Can you work these out from the model? Positions are in its coordinate system, mm. Coordinates: 2 decimals unless noted, no trailing zeros. Order: outer loops, then holes, each group sorted by start corner. A loop starts at its lowest first (then second) coordinate and runs counter-clockwise, first axis right, second up. Notation, with made-up numbers: (-11, 41.25) -> (17, 41.25) arc R31 cw to (17, 71.25) -> close; hole circle Ø7 at (50.25, -8). An arc over 180 degrees is marked (long way). Answer in a Markdown table with one row per item. Add a question column.
1. Imagine slicing it at C-C on z = 1.5. State how many separate pieces and enclosed holes the cut face has, plus the area to 3 significant figures.
2. If I drill on line 1 along Y through (x, z) = (-21, 3.5); line 2 along Y through (x, z) = (-10.5, 5); line 3 along Y through (x, z) = (-76.2, 3.75), over which ranges is the centre line in solid material (lowest first)? Write a range as [from, to].
3. We'd pull the mould along X, two halves only. Please class faces 1 (the face through (-62.396, 55.247, 3.131)), 2 (the face through (-77.12, 137.48, 3.13)), 3 (the face through (66, 42, 0)): pulls with the +X half, pulls with the -X half, needs draft (parallel to the pull), parting line crosses it, or undercut.
4. Imagine slicing it at B-B on x = -127.5. Write out the boundary of the cut face in (y, z).
5. Imagine slicing it at A-A on y = -132.5. Write out the boundary of the cut face in (x, z), plus the area to 3 significant figures.
6. Will these pins go through, and if not, where does the flat tip stop? pin 1 (3 mm diameter, centred on y = -74.5, z = 5, fed in from +X); pin 2 (3 mm diameter, centred on y = 6, z = 2.5, fed in from +X); pin 3 (1.5 mm diameter, centred on x = 40, z = 0.5, fed in from +Y).
from build123d import *

# Parameters (mm, degrees)
F0_W        = 6.35
F0_H        = 50.8
F0_R        = 1.5875
F1_DEPTH    = 6.35
F4_DEPTH    = 6.35
F5_T1_DEPTH = 6.35
F6_R        = 5.08
F7_COUNT    = 3


# Not quite as in the source:
# - a fillet or chamfer that OpenCascade refuses, or shapes differently, is made with other operations: its cross-section is extruded or revolved along the edge and cut away or added
# - a feature of the source that left no trace in its solid (it failed there, or was rolled back) is left out


with BuildPart() as f1:
    # F0 (on Top) → F1 (new body)
    with BuildSketch(Plane.XY):
        with Locations((-76.2, 0)):
            Rectangle(F0_W, F0_H)
        with Locations((-76.2, -19.05)):
            Circle(F0_R, mode=Mode.SUBTRACT)
        with Locations((-76.2, 19.05)):
            Circle(F0_R, mode=Mode.SUBTRACT)
    extrude(amount=F1_DEPTH)



with BuildPart() as f1b:
    # F0 (on Top) → F1, piece 2 (new body)
    with BuildSketch(Plane.XY):
        with Locations((-152.4, 0)):
            Rectangle(F0_W, F0_H)
        with Locations((-152.4, -19.05)):
            Circle(F0_R, mode=Mode.SUBTRACT)
        with Locations((-152.4, 19.05)):
            Circle(F0_R, mode=Mode.SUBTRACT)
    extrude(amount=F1_DEPTH)


with BuildPart() as f1_1:
    add(f1.part)

    add(f1b.part)  # F4 merges F1b
    # F3 (on Top) → F4 (join)
    with BuildSketch(Plane.XY):
        with BuildLine():
            ThreePointArc((31.2797741547, 148.1041402319), (37.4651836805, 146.6615854162), (43.584633363, 144.9608235339))
            ThreePointArc((43.584633363, 144.9608235339), (48.1238684074, 143.5177825724), (52.6154547439, 141.9326408797))
            Line((52.6154547439, 141.9326408797), (55.7904547439, 147.4319021938))
            ThreePointArc((55.7904547439, 147.4319021938), (-78.8174165794, 136.5157700368), (-155.575, 25.4))
            Line((-155.575, 25.4), (-149.225, 25.4))
            ThreePointArc((-149.225, 25.4), (-148.3519798062, 30.0823987171), (-147.3320724153, 34.7350120599))
            ThreePointArc((-147.3320724153, 34.7350120599), (-145.7452505699, 40.8849918834), (-143.9018349238, 46.9629910733))
            ThreePointArc((-143.9018349238, 46.9629910733), (-120.5170928624, 91.5908890283), (-83.7806024253, 126.0716910423))
            ThreePointArc((-83.7806024253, 126.0716910423), (-75.6856337507, 131.0913630593), (-67.2909859281, 135.5919755658))
            ThreePointArc((-67.2909859281, 135.5919755658), (-19.0614902225, 150.1663085232), (31.2797741547, 148.1041402319))
        make_face()
        with BuildLine():
            ThreePointArc((8.2856324479, 82.9270698864), (11.4388872215, 82.551211282), (14.5755338083, 82.0554960938))
            Line((14.5755338083, 82.0554960938), (43.584633363, 144.9608235339))
            ThreePointArc((43.584633363, 144.9608235339), (37.4651836805, 146.6615854162), (31.2797741547, 148.1041402319))
            Line((31.2797741547, 148.1041402319), (8.2856324479, 82.9270698864))
        make_face()
        with BuildLine():
            ThreePointArc((-44.3888773768, 70.534943044), (-41.6699850762, 72.1745313026), (-38.8906138422, 73.7093669758))
            Line((-38.8906138422, 73.7093669758), (-67.2909859281, 135.5919755658))
            ThreePointArc((-67.2909859281, 135.5919755658), (-75.6856337507, 131.0913630593), (-83.7806024253, 126.0716910423))
            Line((-83.7806024253, 126.0716910423), (-44.3888773768, 70.534943044))
        make_face()
        with BuildLine():
            Line((-147.3320724153, 34.7350120599), (-77.2106727023, 31.3697728054))
            ThreePointArc((-77.2106727023, 31.3697728054), (-75.9595282254, 34.2884921917), (-74.5980976675, 37.1574279168))
            Line((-74.5980976675, 37.1574279168), (-143.9018349238, 46.9629910733))
            ThreePointArc((-143.9018349238, 46.9629910733), (-145.7452505699, 40.8849918834), (-147.3320724153, 34.7350120599))
        make_face()
        with BuildLine():
            ThreePointArc((-73.025, 25.4), (-38.6581512265, 66.957882051), (14.5154547439, 75.9415051114))
            Line((14.5154547439, 75.9415051114), (17.6904547439, 81.4407664254))
            ThreePointArc((17.6904547439, 81.4407664254), (16.1359219586, 81.762966235), (14.5755338083, 82.0554960938))
            ThreePointArc((14.5755338083, 82.0554960938), (11.4388872215, 82.551211282), (8.2856324479, 82.9270698864))
            ThreePointArc((8.2856324479, 82.9270698864), (-15.9814809475, 81.7932936843), (-38.8906138422, 73.7093669758))
            ThreePointArc((-38.8906138422, 73.7093669758), (-41.6699850762, 72.1745313026), (-44.3888773768, 70.534943044))
            ThreePointArc((-44.3888773768, 70.534943044), (-61.7898833675, 55.9246004763), (-74.5980976675, 37.1574279168))
            ThreePointArc((-74.5980976675, 37.1574279168), (-75.9595282254, 34.2884921917), (-77.2106727023, 31.3697728054))
            ThreePointArc((-77.2106727023, 31.3697728054), (-78.3497145543, 28.4055074635), (-79.375, 25.4))
            Line((-79.375, 25.4), (-73.025, 25.4))
        make_face()
    extrude(amount=F4_DEPTH)

    # F5: fillet of radius 7.62 on 12 edges, made by hand

    # F5_s2 → F5_t1 (join)
    with BuildSketch(Plane.XY):
        with BuildLine():
            ThreePointArc((-90.1475782146, 121.6004719031), (-84.410893045, 123.0042579182), (-79.3942694829, 119.8875834167))
            Line((-79.3942694829, 119.8875834167), (-83.7806024253, 126.0716910423))
            ThreePointArc((-83.7806024253, 126.0716910423), (-86.9928212861, 123.8769941098), (-90.1475782146, 121.6004719031))
        make_face()
        with BuildLine():
            ThreePointArc((-134.6146538369, 45.648977655), (-140.1386521152, 49.370669263), (-140.6262545751, 56.0135443368))
            ThreePointArc((-140.6262545751, 56.0135443368), (-142.3359988094, 51.5143093511), (-143.9018349238, 46.9629910733))
            Line((-143.9018349238, 46.9629910733), (-134.6146538369, 45.648977655))
        make_face()
        with BuildLine():
            ThreePointArc((-79.8602845165, 37.90195783), (-75.4541334055, 38.5971573414), (-72.1920699233, 41.6395925194))
            ThreePointArc((-72.1920699233, 41.6395925194), (-73.4292909895, 39.4168726535), (-74.5980976675, 37.1574279168))
            Line((-74.5980976675, 37.1574279168), (-79.8602845165, 37.90195783))
        make_face()
        with BuildLine():
            ThreePointArc((-48.8418760227, 76.8130398608), (-47.5248753854, 71.2518102655), (-50.4448624125, 66.3390268333))
            ThreePointArc((-50.4448624125, 66.3390268333), (-47.463259252, 68.50393891), (-44.3888773768, 70.534943044))
            Line((-44.3888773768, 70.534943044), (-48.8418760227, 76.8130398608))
        make_face()
        with BuildLine():
            ThreePointArc((-32.2288512937, 76.8560457563), (-37.9434400628, 76.7836545282), (-42.10110585, 80.7048253346))
            Line((-42.10110585, 80.7048253346), (-38.8906138422, 73.7093669758))
            ThreePointArc((-38.8906138422, 73.7093669758), (-35.5945217294, 75.3563577136), (-32.2288512937, 76.8560457563))
        make_face()
        with BuildLine():
            ThreePointArc((2.7684553264, 83.2939750529), (7.3191534676, 84.6172910948), (10.2074987686, 88.3746146557))
            Line((10.2074987686, 88.3746146557), (8.2856324479, 82.9270698864))
            ThreePointArc((8.2856324479, 82.9270698864), (5.5300876106, 83.1562911392), (2.7684553264, 83.2939750529))
        make_face()
        with BuildLine():
            ThreePointArc((22.2329863038, 149.7296061072), (27.6412349333, 146.1237556106), (28.2996981684, 139.6570920806))
            Line((28.2996981684, 139.6570920806), (31.2797741547, 148.1041402319))
            ThreePointArc((31.2797741547, 148.1041402319), (26.7687208847, 148.9855570423), (22.2329863038, 149.7296061072))
        make_face()
        with BuildLine():
            ThreePointArc((-64.1285580958, 128.7012459955), (-64.3193656083, 134.6041066922), (-60.2353086729, 138.870328775))
            ThreePointArc((-60.2353086729, 138.870328775), (-63.7842132005, 137.2764902356), (-67.2909859281, 135.5919755658))
            Line((-67.2909859281, 135.5919755658), (-64.1285580958, 128.7012459955))
        make_face()
        with BuildLine():
            ThreePointArc((-148.71471153, 28.234645377), (-145.9460574533, 32.7973396391), (-140.8631663364, 34.4245588066))
            Line((-140.8631663364, 34.4245588066), (-147.3320724153, 34.7350120599))
            ThreePointArc((-147.3320724153, 34.7350120599), (-148.0590701809, 31.4924175344), (-148.71471153, 28.234645377))
        make_face()
        with BuildLine():
            ThreePointArc((-86.5356054314, 31.8172913917), (-81.8153136869, 29.8806795078), (-79.375, 25.4))
            ThreePointArc((-79.375, 25.4), (-78.3497145543, 28.4055074635), (-77.2106727023, 31.3697728054))
            Line((-77.2106727023, 31.3697728054), (-86.5356054314, 31.8172913917))
        make_face()
        with BuildLine():
            ThreePointArc((40.7477165489, 138.8090579205), (44.6975181874, 142.6354540642), (50.194139768, 142.8068939441))
            ThreePointArc((50.194139768, 142.8068939441), (46.901752906, 143.9218058508), (43.584633363, 144.9608235339))
            Line((43.584633363, 144.9608235339), (40.7477165489, 138.8090579205))
        make_face()
        with BuildLine():
            ThreePointArc((17.6904547439, 81.4407664254), (16.7569695627, 84.8394313215), (17.4527300656, 88.294606423))
            Line((17.4527300656, 88.294606423), (14.5755338083, 82.0554960938))
            ThreePointArc((14.5755338083, 82.0554960938), (16.1359219586, 81.762966235), (17.6904547439, 81.4407664254))
        make_face()
    extrude(amount=F5_T1_DEPTH)

    # F6
    f6_edges = [f1_1.edges().sort_by_distance(p)[0] for p in [
        (-79.375, 25.4, 3.175),
    ]]
    fillet(f6_edges, radius=F6_R)

    # F7: F1 ×3 about axis
    f7_axis = Axis((0, 0, 0), (0, 0, 1))


with BuildPart() as f1_2:
    add(f1_1.part)
    for i in range(1, F7_COUNT):
        add(f1_1.part.rotate(f7_axis, i * 360 / F7_COUNT))


solid = f1_2.part
Answers follow:
| question | item | result |
|---|---|---|
| 1 | separate pieces | 1 |
| 1 | enclosed holes | 22 |
| 1 | area | 16,000 mm² |
| 2 | line 1 | y = [-156.23, -149.91], [-80.65, -74.41], [74.41, 80.65], [149.91, 156.23] |
| 2 | line 2 | y = [-157.28, -151.01], [-82.68, -76.6], [76.6, 82.68], [151.01, 157.28] |
| 2 | line 3 | y = [-137.99, -115.38], [-36.38, -20.64], [-17.46, 17.46], [20.64, 38.28], [115.38, 137.99] |
| 3 | face 1 | undercut |
| 3 | face 2 | parting line crosses it |
| 3 | face 3 | needs draft |
| 4 | outline | (-92.7, 0) -> (-81.59, 0) -> (-81.59, 6.35) -> (-92.7, 6.35) -> close; (-43.9, 0) -> (-32.92, 0) -> (-32.92, 6.35) -> (-43.9, 6.35) -> close; (33.78, 0) -> (44.64, 0) -> (44.64, 6.35) -> (33.78, 6.35) -> close; (81.59, 0) -> (92.7, 0) -> (92.7, 6.35) -> (81.59, 6.35) -> close |
| 5 | outline | (-85.4, 0) -> (-64.8, 0) -> (-64.8, 6.35) -> (-85.4, 6.35) -> close; (24.99, 0) -> (37.17, 0) -> (37.17, 6.35) -> (24.99, 6.35) -> close; (68.95, 0) -> (81.65, 0) -> (81.65, 6.35) -> (68.95, 6.35) -> close |
| 5 | area | 289 mm² |
| 6 | pin 1 | stops at x = 139.71 |
| 6 | pin 2 | stops at x = 157.57 |
| 6 | pin 3 | stops at y = 152.67 |
